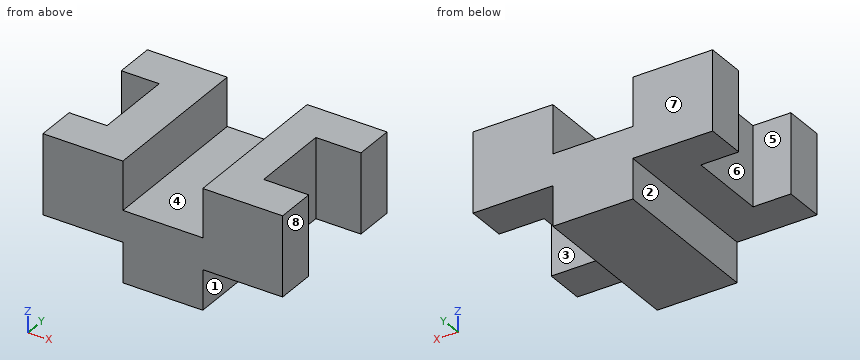
```python
from build123d import *

# Parameters (mm, degrees)
CROQUIS1_W              = 60
CROQUIS1_H              = 30
SALIENTE_EXTRUIR2_DEPTH = 40
CROQUIS2_W              = 20
CROQUIS2_H              = 12.153687435
CORTAR_EXTRUIR1_DEPTH   = 41
CROQUIS3_W              = 20
CROQUIS3_H              = 10
CORTAR_EXTRUIR2_DEPTH   = 41
CROQUIS4_W              = 20
CROQUIS4_H              = 10
CORTAR_EXTRUIR3_DEPTH   = 41
CROQUIS5_W              = 11.276599724
CROQUIS5_H              = 20
CORTAR_EXTRUIR4_DEPTH   = 40
CROQUIS6_W              = 9.488499603
CROQUIS6_H              = 20
CORTAR_EXTRUIR5_DEPTH   = 40


with BuildPart() as part:
    # Croquis1 → Saliente-Extruir2 (new body)
    with BuildSketch(Plane(origin=(0, 0, 0), x_dir=(1, 0, 0), z_dir=(0, 1, 0))):
        Rectangle(CROQUIS1_W, CROQUIS1_H)
    extrude(amount=SALIENTE_EXTRUIR2_DEPTH)

    # Croquis2 → Cortar-Extruir1 (cut, through all)
    with BuildSketch(Plane(origin=(0, 40, 0), x_dir=(1, 0, 0), z_dir=(0, 1, 0))):
        with Locations((0, -8.923156283)):
            Rectangle(CROQUIS2_W, CROQUIS2_H)
    extrude(amount=-CORTAR_EXTRUIR1_DEPTH, mode=Mode.SUBTRACT)

    # Croquis3 → Cortar-Extruir2 (cut, through all)
    with BuildSketch(Plane(origin=(0, 40, 0), x_dir=(1, 0, 0), z_dir=(0, 1, 0))):
        with Locations((-20, 10)):
            Rectangle(CROQUIS3_W, CROQUIS3_H)
    extrude(amount=-CORTAR_EXTRUIR2_DEPTH, mode=Mode.SUBTRACT)

    # Croquis4 → Cortar-Extruir3 (cut, through all)
    with BuildSketch(Plane(origin=(0, 40, 0), x_dir=(1, 0, 0), z_dir=(0, 1, 0))):
        with Locations((20, 10)):
            Rectangle(CROQUIS4_W, CROQUIS4_H)
    extrude(amount=-CORTAR_EXTRUIR3_DEPTH, mode=Mode.SUBTRACT)

    # Croquis5 → Cortar-Extruir4 (cut)
    with BuildSketch(Plane.XY.offset(15)):
        with Locations((24.361700138, 20)):
            Rectangle(CROQUIS5_W, CROQUIS5_H)
    extrude(amount=-CORTAR_EXTRUIR4_DEPTH, mode=Mode.SUBTRACT)

    # Croquis6 → Cortar-Extruir5 (cut)
    with BuildSketch(Plane.XY.offset(15)):
        with Locations((-25.255750199, 20)):
            Rectangle(CROQUIS6_W, CROQUIS6_H)
    extrude(amount=-CORTAR_EXTRUIR5_DEPTH, mode=Mode.SUBTRACT)


solid = part.part
```
Geometry: final body of the model. Coordinates: model frame, mm. Face numbers are marked on the shaded views. A direction names the side the tool comes from. Coordinates: 2 decimals unless noted, no trailing zeros. Order: outer loops, then holes, each group sorted by start corner. A loop starts at its lowest first (then second) coordinate and runs counter-clockwise, first axis right, second up.
Item 1: Material intervals for line 1 along Y through (x, z) = (25, 3); line 2 along X through (y, z) = (3, 13.5); line 3 along Z through (x, y) = (15, 11), sorted ascending.
Answer:
line 1: y = 0 to 10, 30 to 40
line 2: x = -30 to -10, 10 to 30
line 3: z = -5 to 15
Item 2: Contact query for flat-ended pins moving along their axis: P1, Ø1, axis at x = -2.5, y = 20, coming from the +Z side; P2, Ø1, axis at x = -20, z = -2, coming from the -Y side; P3, Ø13.5, axis at y = 20.5, z = 7.5, coming from the -X side; P4, Ø5, axis at y = 15, z = -11.5, coming from the -X side. Output: stop coordinate, or through.
Answer:
P1: stops at z = 2.85
P2: stops at y = 0
P3: stops at x = -20.51
P4: stops at x = -10
Item 3: Draft query along Y for the marked faces 6, 7 and 8. Return one class per face: released by +Y, released by -Y, zero draft, split by the parting line, or undercut.
Answer:
face 6: undercut
face 7: released by +Y
face 8: zero draft
Item 4: Access query for the marked faces 1, 2, 3, 4 and 5. Directions: +Z, -Z, +X, -X, +Y, -Y. A direction counts if a zero-diameter tool reaches every point of the face in a straight line with its end or side. Return the directions, or none.
Answer:
face 1: -Z, +X, +Y, -Y
face 2: -Z, -X, +Y, -Y
face 3: +Z, -Z, +X
face 4: +Z, +Y, -Y
face 5: +Z, -Z, -X
Item 5: Section query C-C (y = 28). Output: boundary loops of the cut face in (x, z).
Answer:
outline: (-20.51, -5) - (-10, -5) - (-10, -15) - (10, -15) - (10, -5) - (18.72, -5) - (18.72, 15) - (10, 15) - (10, 2.85) - (-10, 2.85) - (-10, 15) - (-20.51, 15) - close
Item 6: Section query D-D (z = -1). Output: boundary loops of the cut face in (x, y), then the cut area to 3 significant figures.
Answer:
outline: (-30, 0) - (30, 0) - (30, 10) - (18.72, 10) - (18.72, 30) - (30, 30) - (30, 40) - (-30, 40) - (-30, 30) - (-20.51, 30) - (-20.51, 10) - (-30, 10) - close
area: 1,980 mm2
Item 7: Section query B-B (z = 10). Output: boundary loops of the cut face in (x, y).
Answer:
outline: (-30, 0) - (-10, 0) - (-10, 40) - (-30, 40) - (-30, 30) - (-20.51, 30) - (-20.51, 10) - (-30, 10) - close; (10, 0) - (30, 0) - (30, 10) - (18.72, 10) - (18.72, 30) - (30, 30) - (30, 40) - (10, 40) - close
Item 8: Section query A-A (x = 26). Output: boundary loops of the cut face in (y, z).
Answer:
outline: (0, -5) - (10, -5) - (10, 15) - (0, 15) - close; (30, -5) - (40, -5) - (40, 15) - (30, 15) - close
